Job drawing, mm, ordinate dimensions from the low corner. One solid piece. Round coordinates to 2 decimals unless told otherwise and drop trailing zeros. Loops run counter-clockwise (first coordinate to the right, second up) from the corner with the lowest first, then second, coordinate; pieces in that order, holes last. Notation, with made-up numbers: (-6, 63.25) - (41, 63.25) arc R28 cw to (41, 92.25) - close; hole circle Ø8 at (-27.75, 76). An arc over 180 degrees is marked (long way). Answer as CSV lines item,"result". Start each with the question number.
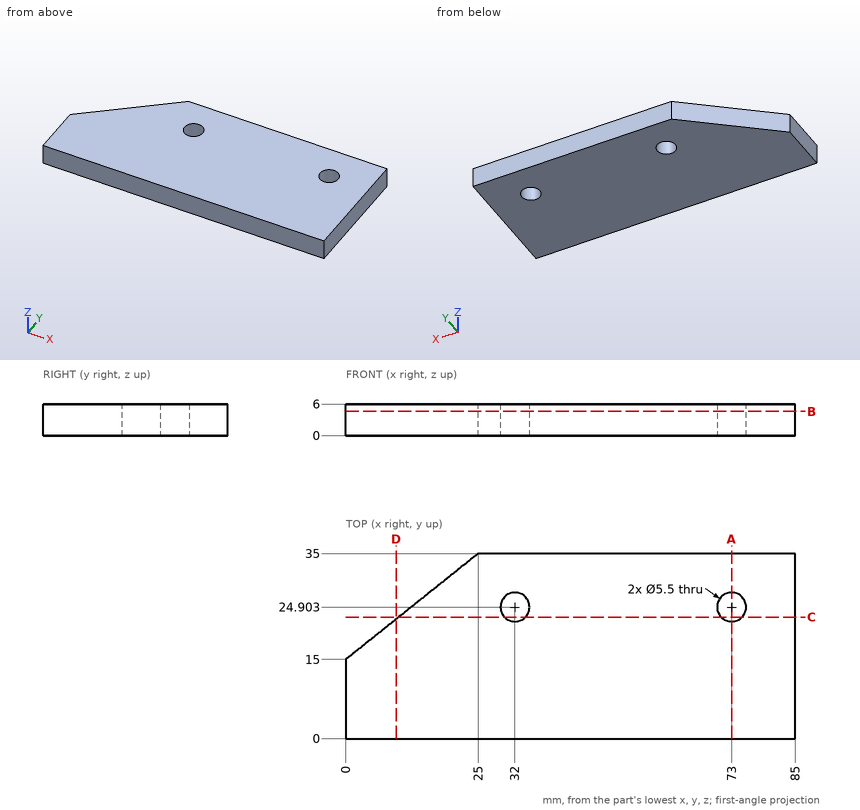
Q1. Band-saw the part on C-C, the plane y = 23. List the corners of the cut face in (x, z) (1 decimal).
Q2. Pin check, flat tip, straight feed: pin 1 Ø2 at (y, z) = (18.5, 2) entering from -X (1 decimal). Stop position of the tip, or through.
Q3. Band-saw the part on B-B, the plane z = 4.6. List the corners of the cut face in (x, y).
Q4. Band-saw the part on A-A, the plane x = 73. List the corners of the cut face in (y, z), then the cut area to 3 significant figures.
Q5. Band-saw the part on D-D, the plane x = 9.5. List the corners of the cut face in (y, z), then the cut area to 3 significant figures.
Q6. Wall check: probe 1 along Y at (x, z) = (32, 3.05); probe 2 along X at (y, z) = (24.5, 1.6) (1 decimal); probe 3 along Y at (x, z) = (16.5, 5.1). Give the ranges that are in metal, low to high. Write a range as [from, to].
Reported:
1,outline,"(10, 0) - (30, 0) - (30, 6) - (10, 6) - close; (34, 0) - (71, 0) - (71, 6) - (34, 6) - close; (75, 0) - (85, 0) - (85, 6) - (75, 6) - close"
2,pin 1,"stops at x = 3.1"
3,outline,"(0, 0) - (85, 0) - (85, 35) - (25, 35) - (0, 15) - close; hole circle Ø5.5 at (32, 24.9); hole circle Ø5.5 at (73, 24.9)"
4,outline,"(0, 0) - (22.15, 0) - (22.15, 6) - (0, 6) - close; (27.65, 0) - (35, 0) - (35, 6) - (27.65, 6) - close"
4,area,"177 mm2"
5,outline,"(0, 0) - (22.6, 0) - (22.6, 6) - (0, 6) - close"
5,area,"136 mm2"
6,probe 1,"y = [0, 22.15], [27.65, 35]"
6,probe 2,"x = [11.9, 29.3], [34.7, 70.3], [75.7, 85]"
6,probe 3,"y = [0, 28.2]"
